Read the model definition and answer for the solid it produces. Units are mm, in the model's axes. Face numbers are marked on the shaded views. A direction names the side the tool comes from. Round coordinates to 2 decimals unless told otherwise and drop trailing zeros. Write each loop counter-clockwise with the first axis right and the second up, starting at its lowest first coordinate (ties: lowest second). Pieces come first, ordered by that corner, then holes. Notation, with made-up numbers: (-0.75, -4) - (37.25, -4) arc R21 ccw to (37.25, 25) - close; hole circle Ø7 at (34.25, -6.5). An arc over 180 degrees is marked (long way). Answer as CSV lines item,"result". Start each with the question number.
1) Find section B-B on y = -2. Determine the outline of the cut face in (x, z), then the cut area to 3 significant figures.
2) Consider line 1 along X through (y, z) = (2.5, -28); line 2 along Y through (x, z) = (-31.75, 27); line 3 along Y through (x, z) = (-31, -2.5). Determine where each line is inside the solid, lowest interval first.
3) Find section C-C on z = -17. Determine the outline of the cut face in (x, y), then the cut area to 3 significant figures.
4) Find section A-A on x = 31.75. Determine the outline of the cut face in (y, z).
5) Which of the six approach directions +Z, -Z, +X, -X, +Y, -Y give full straight-line access (tool end or side, diameter ignored) to the marked faces 1, 2 and 3?
6) Find section D-D on x = -31.5. Determine the outline of the cut face in (y, z), then the cut area to 3 significant figures.
7) For a pull along Z with two mould halves and no side action, classify the marked faces 4, 5, 6 and 7 as +Z half, -Z half, draft (parallel to the pull), parting line (faces both ways), or undercut.
8) Each of these flat-tipped pins is pushed along its axis until it touches: pin 1 (12 mm diameter, centred on x = 28.5, z = -22.5, fed in from +Y); pin 2 (11.5 mm diameter, centred on x = 27.5, z = 2.5, fed in from -Y); pin 3 (1.5 mm diameter, centred on x = 30, z = -16, fed in from +Y); pin 4 (4 mm diameter, centred on x = 3, z = -14.5, fed in from +Y). Where does it stop, or does it pass through?
Autodesk Inventor part; units mm, degrees
ref_plane "YZ Plane" through (0, 0, 0) normal (1, 0, 0) x (0, 1, 0)
ref_plane "XZ Plane" through (0, 0, 0) normal (0, 1, 0) x (-1, 0, 0)
ref_plane "XY Plane" through (0, 0, 0) normal (0, 0, 1) x (1, 0, 0)
sketch "Sketch1" plane through (0, 0, 0) normal (0, 0, 1) x (1, 0, 0)
  arc A0 (-13.9696, -0.1018) -> (13.9696, -0.1018) centre (0, 0) ccw
  line L0 (0, 64.951) -> (0, -100.8994)
  arc A1 (-23.2558, -13.0558) -> (23.2558, -13.0558) centre (0, 0) ccw
  line L1 (-23.2558, -13.0558) -> (-37.846, -13.0558)
  line L2 (37.846, -13.0558) -> (23.2558, -13.0558)
  arc A2 (-25.6593, 6.2482) -> (-37.846, 5.9942) centre (-31.75, 5.9942) ccw
  line L3 (-37.846, -0.3558) -> (-37.846, 5.9942)
  line L4 (-25.6593, -0.1018) -> (-25.6593, 6.2482)
  arc A3 (37.846, 5.9942) -> (25.6593, 6.2482) centre (31.75, 5.9942) ccw
  line L5 (37.846, -0.3558) -> (37.846, 5.9942)
  line L6 (25.6593, -0.1018) -> (25.6593, 6.2482)
  line L7 (-25.6593, -0.1018) -> (-13.9696, -0.1018)
  line L8 (13.9696, -0.1018) -> (25.6593, -0.1018)
  circle A4 centre (-31.75, 5.9942) radius 3.175
  circle A5 centre (31.75, 5.9942) radius 3.175
  line L9 (-37.846, -0.3558) -> (-37.846, -13.0558)
  line L10 (37.846, -0.3558) -> (37.846, -13.0558)
  dimension "d0" = 27.94
  dimension "d4" = 12.7
  dimension "d5" = 12.192
  dimension "d6" = 63.5
  dimension "d7" = 6.35
  dimension "d8" = 6.35
  dimension "d13" = 12.7
  dimension "d14" = 6.35
  dimension "d29" = 14.5902
  dimension "d31" = 14.5902
  dimension "d32" = 6.35
extrude "Extrusion1" add sketch "Sketch1" along normal mid plane 60.96
sketch "Sketch3" plane through (-25.6593, -0.1018, 30.48) normal (1, 0, 0) x (0, 0, -1)
  line L0 (60.96, 0) -> (0, 0)
  line L1 (60.96, 12.192) -> (0, 12.192)
  line L2 (6.35, 0) -> (54.61, 0)
  line L3 (54.61, 0) -> (54.61, 12.192)
  line L4 (54.61, 12.192) -> (6.35, 12.192)
  line L5 (6.35, 12.192) -> (6.35, 0)
  line L6 (0, 12.192) -> (0, 6.096)
  line L7 (60.96, 6.35) -> (60.96, 12.192)
  point P0 (30.48, 0.1018)
  point P1 (6.35, 12.192)
  dimension "d23" = 6.35
  dimension "d24" = 6.35
extrude "Extrusion3" cut sketch "Sketch3" along normal mid plane 152.4
properties part number "Relaxation chamber outer holder"
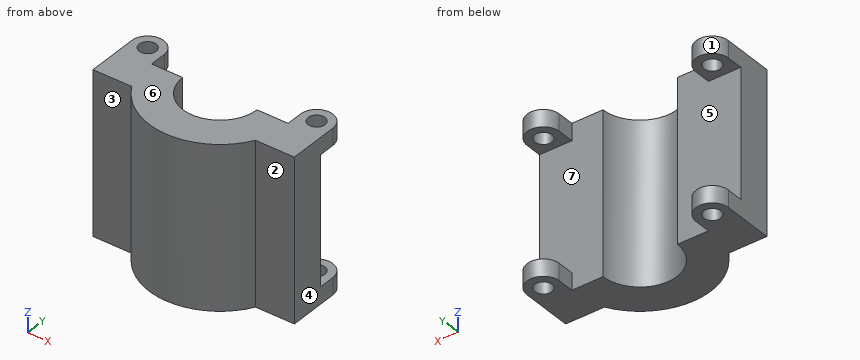
Check values:
1,outline,"(-37.85, -30.48) - (-13.83, -30.48) - (-13.83, 30.48) - (-37.85, 30.48) - close; (13.83, -30.48) - (37.85, -30.48) - (37.85, 30.48) - (13.83, 30.48) - close"
1,area,"2,930 mm^2"
2,line 1,"x = -37.85 to -25.66, 25.66 to 37.85"
2,line 2,"y = -13.06 to 2.82, 9.17 to 12.09"
2,line 3,"y = -13.06 to -0.1"
3,outline,"(-37.85, -13.06) - (-23.26, -13.06) arc R26.67 ccw to (23.26, -13.06) - (37.85, -13.06) - (37.85, -0.1) - (13.97, -0.1) arc R13.97 cw to (-13.97, -0.1) - (-37.85, -0.1) - close"
3,area,"1,130 mm^2"
4,outline,"(-13.06, -30.48) - (2.82, -30.48) - (2.82, -24.13) - (-0.1, -24.13) - (-0.1, 24.13) - (2.82, 24.13) - (2.82, 30.48) - (-13.06, 30.48) - close; (9.17, -30.48) - (12.09, -30.48) - (12.09, -24.13) - (9.17, -24.13) - close; (9.17, 24.13) - (12.09, 24.13) - (12.09, 30.48) - (9.17, 30.48) - close"
5,face 1,"+Z, -Z, +Y"
5,face 2,"+Z, -Z, +X, -Y"
5,face 3,"+Z, -Z, -X, -Y"
6,outline,"(-13.06, -30.48) - (2.83, -30.48) - (2.83, -24.13) - (-0.1, -24.13) - (-0.1, 24.13) - (2.83, 24.13) - (2.83, 30.48) - (-13.06, 30.48) - close; (9.16, -30.48) - (12.09, -30.48) - (12.09, -24.13) - (9.16, -24.13) - close; (9.16, 24.13) - (12.09, 24.13) - (12.09, 30.48) - (9.16, 30.48) - close"
6,area,"864 mm^2"
7,face 4,"draft"
7,face 5,"undercut"
7,face 6,"+Z half"
7,face 7,"undercut"
8,pin 1,"stops at y = 12.09"
8,pin 2,"stops at y = -15.43"
8,pin 3,"stops at y = -0.1"
8,pin 4,"stops at y = -13.04"
